from build123d import *

# Parameters (mm, degrees)
SKIZZE2_W                       = 15
SKIZZE2_H                       = 7
AUFSATZ_LINEAR_AUSTRAGEN1_DEPTH = 1
SKIZZE3_R                       = 2.25
SKIZZE3_R_2                     = 1
AUFSATZ_LINEAR_AUSTRAGEN2_DEPTH = 15
SCHNITT_LINEAR_AUSTRAGEN1_DEPTH = 5
LINEARES_MUSTER1_COUNT          = 2
LINEARES_MUSTER1_PITCH          = 10
SKIZZE7_W                       = 5.129171307
SKIZZE7_H                       = 1
VERBREITERUNG_DEPTH             = 2.5
FASE1_SIZE                      = 0.5
AUFSATZ_LINEAR_AUSTRAGEN3_DEPTH = 5


with BuildPart() as part:
    # Skizze2 → Aufsatz-Linear austragen1 (new body)
    with BuildSketch(Plane(origin=(0, 0, 0), x_dir=(1, 0, 0), z_dir=(0, 1, 0))):
        Rectangle(SKIZZE2_W, SKIZZE2_H)
    extrude(amount=AUFSATZ_LINEAR_AUSTRAGEN1_DEPTH)

    # Skizze3 → Aufsatz-Linear austragen2 (add)
    with BuildSketch(Plane(origin=(7.5, 0, 0), x_dir=(0, 0, -1), z_dir=(1, 0, 0))):
        with Locations((-3.5, 2.25)):
            Circle(SKIZZE3_R)
        with Locations((-3.5, 2.25)):
            Circle(SKIZZE3_R_2, mode=Mode.SUBTRACT)
    extrude(amount=-AUFSATZ_LINEAR_AUSTRAGEN2_DEPTH)

    # Skizze5 → Schnitt-Linear austragen1 (cut)
    with BuildSketch(Plane(origin=(7.5, 0, 0), x_dir=(0, 0, -1), z_dir=(1, 0, 0))):
        with BuildLine():
            Line((-1.629171307, 1), (-1.629171307, 0))
            Line((-1.629171307, 0), (-3.5, 0))
            ThreePointArc((-3.5, 0), (-4.560660172, 4.234313483), (-1.629171307, 1))
        make_face()
    schnitt_linear_austragen1 = extrude(amount=-SCHNITT_LINEAR_AUSTRAGEN1_DEPTH, mode=Mode.SUBTRACT)

    # Lineares Muster1: Schnitt-Linear austragen1 ×2
    with Locations(*[(-i * LINEARES_MUSTER1_PITCH, 0, 0) for i in range(1, LINEARES_MUSTER1_COUNT)]):
        add(schnitt_linear_austragen1, mode=Mode.SUBTRACT)

    # Skizze7 → Verbreiterung (add)
    with BuildSketch(Plane(origin=(7.5, 0, 0), x_dir=(0, 0, -1), z_dir=(1, 0, 0))):
        with Locations((0.935414346, 0.5)):
            Rectangle(SKIZZE7_W, SKIZZE7_H)
    verbreiterung = extrude(amount=VERBREITERUNG_DEPTH)

    # Spiegeln1: Verbreiterung across plane
    add(verbreiterung.mirror(Plane(origin=(0, 0, 0), x_dir=(0, 0, 1), z_dir=(1, 0, 0))))

    # Fase1
    fase1_edges = [part.edges().sort_by_distance(p)[0] for p in [
        (2.5, 2.25, 4.5),
        (-2.5, 2.25, 4.5),
    ]]
    chamfer(fase1_edges, length=FASE1_SIZE)

    # Skizze9 → Aufsatz-Linear austragen3 (add)
    with BuildSketch(Plane(origin=(2.5, 0, 0), x_dir=(0, 0, -1), z_dir=(1, 0, 0))):
        Polygon((-1.629171307, 1), (3.5, 1), (-2.423928807, 4.225998681), align=None)
    extrude(amount=-AUFSATZ_LINEAR_AUSTRAGEN3_DEPTH)


solid = part.part
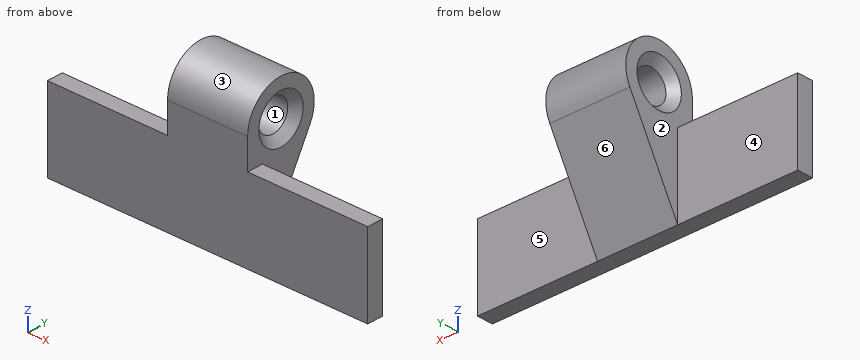
Design review of the part built by this model. Coordinates are the model's own, in mm. Face numbers are marked on the shaded views. A direction names the side the tool comes from. Give positions to 0.01 mm unless a question says otherwise; leave off trailing zeros. Write each loop counter-clockwise with the first axis right and the second up, starting at its lowest first coordinate (ties: lowest second). Pieces come first, ordered by that corner, then holes. Notation, with made-up numbers: M 73.5,-6 L 88.5,-6 A31 ccw 88.5,25 Z; hole C 43.5,1 d3. An arc over 180 degrees is marked long. Answer as a JSON object with one key per item and string values. Group by question number.
1) We need section D-D (y = 4). Give the boundary of the cut face in (x, z).
2) We need section A-A (y = 2.25). Give the boundary of the cut face in (x, z), and give its area (3 significant figures).
3) Tool access review of the marked faces 4, 5 and 6: name each direction out of +Z, -Z, +X, -X, +Y, -Y from which nothing blocks a thin tool from reaching the whole face with its end or side.
4) For line 1 along Y through (x, z) = (-0.7, 3.5); line 2 along Z through (x, y) = (1.5, 1.7); line 3 along X through (y, z) = (2.5, 0.5), list the stretches that pass through material, from the lowest coordinate up.
5) We need section B-B (z = 1.25). Give the boundary of the cut face in (x, y), and give its area (3 significant figures).
6) We need section C-C (x = -8.25). Give the boundary of the cut face in (y, z), and give its area (3 significant figures).
7) Clearance check with flat-ended pins moving along their axes: pin 1 Ø1.1 at (x, y) = (-7, 0.5) entering from +Z; pin 2 Ø2.5 at (y, z) = (2.25, 3.5) entering from -X; pin 3 Ø1.5 at (x, z) = (-5, -1.5) entering from +Y. State where each tip first meets the part, or that it passes through.
8) Mouldability with a two-part tool opening along Z and no side actions: class the marked faces 1, 2 and 3 as released by +Z, released by -Z, zero draft, split by the parting line, or undercut.
Answer key:
{
 "1": {"outline": "M -2.5,2.01 L 2.5,2.01 L 2.5,4.91 L -2.5,4.91 Z"},
 "2": {"outline": "M -2.5,-1.2 L 2.5,-1.2 L 2.5,2 L 2,2.5 L -2,2.5 L -2.5,2 Z; M -2.5,5 L -2,4.5 L 2,4.5 L 2.5,5 L 2.5,5.75 L -2.5,5.75 Z", "area": "24.3 mm²"},
 "3": {"face 4": "+Z, -Z, -X, +Y", "face 5": "+Z, -Z, +X, +Y", "face 6": "-Z, +X, -X, +Y"},
 "4": {"line 1": "y = 0 to 1.25, 3.25 to 4.5", "line 2": "z = -2.21 to 2.66, 4.34 to 5.68", "line 3": "x = -2.5 to 2.5"},
 "5": {"outline": "M -10,0 L 10,0 L 10,1 L 2.5,1 L 2.5,3.59 L -2.5,3.59 L -2.5,1 L -10,1 Z", "area": "32.9 mm²"},
 "6": {"outline": "M 0,-3.5 L 1,-3.5 L 1,1.63 L 0,1.63 Z", "area": "5.13 mm²"},
 "7": {"pin 1": "stops at z = 1.63", "pin 2": "stops at x = -2.25", "pin 3": "stops at y = 1"},
 "8": {"face 1": "undercut", "face 2": "zero draft", "face 3": "split by the parting line"}
}
